```python
from build123d import *

# Parameters (mm, degrees)
SKETCH_R        = 1.875
SKETCH_W        = 26.28
SKETCH_H        = 35.8
SKETCH_W_2      = 34.45
SKETCH_W_3      = 44.27
PAD_DEPTH       = 3
SKETCH001_W     = 6
SKETCH001_H     = 3
PAD001_DEPTH    = 7
SKETCH002_W     = 3
SKETCH002_H     = 7
PAD002_DEPTH    = 4.5
SKETCH003_W     = 7
SKETCH003_H     = 2
PAD003_DEPTH    = 6
SKETCH004_R     = 2
POCKET_DEPTH    = 5
SKETCH005_R     = 5
SKETCH005_R_2   = 1.875
PAD004_DEPTH    = 6
POCKET001_DEPTH = 2.25
CHAMFER_SIZE    = 2.5
SKETCH007_W     = 46.28
SKETCH007_H     = 5
SKETCH007_W_2   = 18
SKETCH007_H_2   = 7
SKETCH007_W_3   = 10
SKETCH007_H_3   = 6
POCKET002_DEPTH = 2.1


with BuildPart() as part:
    # Sketch → Pad (new body)
    with BuildSketch(Plane.XY):
        with BuildLine():
            Line((-72.5, 50.8), (-72.5, -49.125249))
            Line((-72.5, -49.125249), (-40.543855, -50.8))
            Line((-40.543855, -50.8), (-35.113855, -50.8))
            ThreePointArc((-35.113855, -50.8), (-31.221817, -52.647375), (-27.328445, -50.802814))
            Line((-27.328445, -50.802814), (-16.628445, -50.802814))
            Line((-16.628445, -50.802814), (-8.628445, -50.8))
            Line((-8.628445, -50.8), (9.371555, -50.8))
            ThreePointArc((9.371555, -50.8), (13.23, -52.62), (17.088445, -50.8))
            Line((17.088445, -50.8), (72.5, -50.8))
            Line((72.5, -50.8), (72.5, 50.8))
            Line((49.5, 50.8), (72.5, 50.8))
            Line((49.5, 50.8), (49.5, 61.8))
            Line((49.5, 61.8), (-62.5, 61.8))
            Line((-62.5, 50.8), (-62.5, 61.8))
            Line((-72.5, 50.8), (-62.5, 50.8))
        make_face()
        with Locations((13.23, 47.62)):
            Circle(SKETCH_R, mode=Mode.SUBTRACT)
        with Locations((13.23, -47.62)):
            Circle(SKETCH_R, mode=Mode.SUBTRACT)
        with Locations((-31.22, -47.62)):
            Circle(SKETCH_R, mode=Mode.SUBTRACT)
        with Locations((-31.22, 47.62)):
            Circle(SKETCH_R, mode=Mode.SUBTRACT)
        with Locations((-49.36, 22.9)):
            Rectangle(SKETCH_W, SKETCH_H, mode=Mode.SUBTRACT)
        with Locations((-8.995, 22.9)):
            Rectangle(SKETCH_W_2, SKETCH_H, mode=Mode.SUBTRACT)
        with Locations((40.365, 22.9)):
            Rectangle(SKETCH_W_3, SKETCH_H, mode=Mode.SUBTRACT)
        with Locations((40.365, -22.9)):
            Rectangle(SKETCH_W_3, SKETCH_H, mode=Mode.SUBTRACT)
        with Locations((-8.995, -22.9)):
            Rectangle(SKETCH_W_2, SKETCH_H, mode=Mode.SUBTRACT)
        with Locations((-49.36, -22.9)):
            Rectangle(SKETCH_W, SKETCH_H, mode=Mode.SUBTRACT)
        with BuildLine():
            ThreePointArc((-45.5, 55.8), (-44, 57.3), (-45.5, 58.8))
            Line((-45.5, 58.8), (-51.901924, 58.8))
            ThreePointArc((-51.901924, 58.8), (-57.5, 57.3), (-51.901924, 55.8))
            Line((-45.5, 55.8), (-51.901924, 55.8))
        make_face(mode=Mode.SUBTRACT)
        with BuildLine():
            ThreePointArc((39.5, 55.8), (41, 57.3), (39.5, 58.8))
            Line((39.5, 58.8), (33.098076, 58.8))
            ThreePointArc((33.098076, 58.8), (27.5, 57.3), (33.098076, 55.8))
            Line((39.5, 55.8), (33.098076, 55.8))
        make_face(mode=Mode.SUBTRACT)
    extrude(amount=PAD_DEPTH)

    # Sketch001 (on Face9 of Pad) → Pad001 (join)
    with BuildSketch(Plane.XZ.offset(50.8)):
        with Locations((41.5, 1.5)):
            Rectangle(SKETCH001_W, SKETCH001_H)
    extrude(amount=PAD001_DEPTH)

    # Sketch002 (on Face56 of Pad001) → Pad002 (join)
    with BuildSketch(Plane.XY.offset(3)):
        with Locations((40, -54.3)):
            Rectangle(SKETCH002_W, SKETCH002_H)
    extrude(amount=PAD002_DEPTH)

    # Sketch003 (on Face61 of Pad002) → Pad003 (join)
    with BuildSketch(Plane(origin=(38.5, 0, 0), x_dir=(0, -1, 0), z_dir=(-1, 0, 0))):
        with Locations((54.3, 6.5)):
            Rectangle(SKETCH003_W, SKETCH003_H)
    extrude(amount=PAD003_DEPTH)

    # Sketch004 (on Face67 of Pad003) → Pocket (cut)
    with BuildSketch(Plane.XY.offset(7.5)):
        with Locations((35.5, -54.8)):
            Circle(SKETCH004_R)
    extrude(amount=-POCKET_DEPTH, mode=Mode.SUBTRACT)

    # Sketch005 → Pad004 (join)
    with BuildSketch(Plane.XY):
        with Locations((-31.22, 47.62)):
            Circle(SKETCH005_R)
        with Locations((-31.22, 47.62)):
            Circle(SKETCH005_R_2, mode=Mode.SUBTRACT)
        with Locations((13.23, 47.62)):
            Circle(SKETCH005_R)
        with Locations((13.23, 47.62)):
            Circle(SKETCH005_R_2, mode=Mode.SUBTRACT)
        with Locations((-31.22, -47.62)):
            Circle(SKETCH005_R)
        with Locations((-31.22, -47.62)):
            Circle(SKETCH005_R_2, mode=Mode.SUBTRACT)
        with Locations((13.23, -47.62)):
            Circle(SKETCH005_R)
        with Locations((13.23, -47.62)):
            Circle(SKETCH005_R_2, mode=Mode.SUBTRACT)
    extrude(amount=PAD004_DEPTH)

    # Sketch006 (on Face5 of Pad004) → Pocket001 (cut)
    with BuildSketch(Plane.XY.offset(3)):
        with BuildLine():
            ThreePointArc((-54.5, 60.68), (-57.88, 57.3), (-54.5, 53.92))
            Line((-54.5, 53.92), (-40.82, 53.92))
            ThreePointArc((-40.82, 53.92), (-37.44, 57.3), (-40.82, 60.68))
            Line((-40.82, 60.68), (-54.5, 60.68))
        make_face()
        with BuildLine():
            ThreePointArc((30.5, 60.84), (26.96, 57.3), (30.5, 53.76))
            Line((30.5, 53.76), (44.52, 53.76))
            ThreePointArc((44.52, 53.76), (48.06, 57.3), (44.52, 60.84))
            Line((44.52, 60.84), (30.5, 60.84))
        make_face()
    extrude(amount=-POCKET001_DEPTH, mode=Mode.SUBTRACT)

    # Chamfer
    chamfer_edges = [part.edges().sort_by_distance(p)[0] for p in [
        (-29.345, -47.62, 1.5),
        (-33.095, -47.62, 0),
        (-33.095, -47.62, 3),
        (15.105, -47.62, 1.5),
        (11.355, -47.62, 0),
        (11.355, -47.62, 3),
        (-29.345, 47.62, 1.5),
        (-33.095, 47.62, 0),
        (-33.095, 47.62, 3),
        (15.105, 47.62, 1.5),
        (11.355, 47.62, 0),
        (11.355, 47.62, 3),
    ]]
    chamfer(chamfer_edges, length=CHAMFER_SIZE)

    # Sketch007 (on Face52 of Pad) → Pocket002 (cut)
    with BuildSketch(Plane(origin=(0, 0, 0), x_dir=(1, 0, 0), z_dir=(0, 0, -1))):
        with Locations((-49.36, -34.3)):
            Rectangle(SKETCH007_W, SKETCH007_H)
        with Locations((-63.5, -44.3)):
            Rectangle(SKETCH007_W_2, SKETCH007_H_2)
        with Locations((-67.5, 25.2)):
            Rectangle(SKETCH007_W_3, SKETCH007_H_3)
    extrude(amount=-POCKET002_DEPTH, mode=Mode.SUBTRACT)


solid = part.part
```
Source: CAD feature listing. Evaluate the final solid. Frame: model axes, mm. A direction names the side the tool comes from. Coordinates: 2 decimals unless noted, no trailing zeros. Write each loop counter-clockwise with the first axis right and the second up, starting at its lowest first coordinate (ties: lowest second). Pieces come first, ordered by that corner, then holes. Notation, with made-up numbers: M 25,84 L 53,84 A8 ccw 53,89 Z; hole C 71,4 d6. An arc over 180 degrees is marked long. Answer as a JSON object with one key per item and string values.
1. Cut plane C-C on x = 35.5. Output: boundary loops of the cut face in (y, z), plus the area to 3 significant figures.
Evaluation:
{"outline": "M -57.8,5.5 L -56.8,5.5 L -56.8,7.5 L -57.8,7.5 Z; M -52.8,5.5 L -50.8,5.5 L -50.8,7.5 L -52.8,7.5 Z; M -50.8,0 L -40.8,0 L -40.8,3 L -50.8,3 Z; M -5,0 L 5,0 L 5,3 L -5,3 Z; M 40.8,0 L 55.8,0 L 55.8,0.75 L 53.76,0.75 L 53.76,3 L 40.8,3 Z; M 58.8,0 L 61.8,0 L 61.8,3 L 60.84,3 L 60.84,0.75 L 58.8,0.75 Z", "area": "111 mm^2"}
2. Cut plane B-B on y = 18.5. Output: boundary loops of the cut face in (x, z), plus the area to 3 significant figures.
Evaluation:
{"outline": "M -72.5,0 L -62.5,0 L -62.5,3 L -72.5,3 Z; M -36.22,0 L -26.22,0 L -26.22,3 L -36.22,3 Z; M 8.23,0 L 18.23,0 L 18.23,3 L 8.23,3 Z; M 62.5,0 L 72.5,0 L 72.5,3 L 62.5,3 Z", "area": "120 mm^2"}
3. Draft query along Y for faces 1 (the flat face through (41.5, -54, 5)), 2 (the flat face through (58, -50.8, 1)), 3 (the flat face through (-47, 40.8, 1)), 4 (the flat face through (62.5, 23, 1)). Return one class per face: released by +Y, released by -Y, zero draft, split by the parting line, or undercut.
Evaluation:
{"face 1": "zero draft", "face 2": "released by -Y", "face 3": "undercut", "face 4": "undercut"}
4. Cut plane D-D on x = 13.23. Output: boundary loops of the cut face in (y, z) (3 decimals).
Evaluation:
{"outline": "M -52.62,0 L -51.995,0 L -49.495,2.5 L -49.495,6 L -52.62,6 Z; M -45.745,2.5 L -43.245,0 L 43.245,0 L 45.745,2.5 L 45.745,6 L 42.62,6 L 42.62,3 L -42.62,3 L -42.62,6 L -45.745,6 Z; M 49.495,2.5 L 51.995,0 L 61.8,0 L 61.8,3 L 52.62,3 L 52.62,6 L 49.495,6 Z"}
5. Access query for faces 5 (the flat face through (-68, -25, 2.1)), 6 (the cylindrical face through (-28.913, 43.184, 4.479)), 7 (the flat face through (18.23, 23, 1)), 8 (the flat face through (36.2, -52.7, 5.5)). Directions: +Z, -Z, +X, -X, +Y, -Y. A direction counts if a zero-diameter tool reaches every point of the face in a straight line with its end or side. Return the directions, or none.
Evaluation:
{"face 5": "-Z, -X", "face 6": "+Z", "face 7": "+Z, -Z", "face 8": "-Z, +Y, -Y"}
6. Ray query, L1, parallel to X at y = 30.5, z = 1.75; L2, parallel to Y at x = 23, z = 1.5; L3, parallel to X at y = 57.3, z = 0.4. Return the intervals inside material, ascending.
Evaluation:
{"L1": "-72.5 to -62.5, -36.22 to -26.22, 8.23 to 18.23, 62.5 to 72.5", "L2": "-50.8 to -40.8, -5 to 5, 40.8 to 61.8", "L3": "-62.5 to -57.5, -44 to 27.5, 41 to 49.5"}
7. Cut plane A-A on x = -31.22. Output: boundary loops of the cut face in (y, z) (3 decimals), plus the area to 3 significant figures.
Evaluation:
{"outline": "M -52.647,0 L -51.995,0 L -49.495,2.5 L -49.495,6 L -52.62,6 L -52.62,3 L -52.647,3 Z; M -45.745,2.5 L -43.245,0 L 31.8,0 L 31.8,2.1 L 36.8,2.1 L 36.8,0 L 43.245,0 L 45.745,2.5 L 45.745,6 L 42.62,6 L 42.62,3 L -42.62,3 L -42.62,6 L -45.745,6 Z; M 49.495,2.5 L 51.995,0 L 61.8,0 L 61.8,3 L 52.62,3 L 52.62,6 L 49.495,6 Z", "area": "335 mm^2"}
8. Contact query for flat-ended pins moving along their axis: P1, Ø0.9, axis at x = -46, z = 2, coming from the -Y side; P2, Ø10, axis at x = 15, y = 26.5, coming from the +Z side; P3, Ø1, axis at x = -68.5, z = 1.5, coming from the +Y side; P4, Ø1.5, axis at x = 13.5, y = -21.5, coming from the -Z side. Output: stop coordinate, or through.
Evaluation:
{"P1": "y = -50.54", "P2": "z = 3", "P3": "y = 50.8", "P4": "z = 0"}
